from build123d import *

# Parameters (mm, degrees)
EXTRUDE_1_DEPTH = 3


with BuildPart() as part:
    # 草圖1 → 填料-伸長1 (new body)
    with BuildSketch(Plane.XY):
        Polygon((0, -10), (30, -10), (30, -40), (40, -40), (40, -10), (40, 0), (0, 0), align=None)
        Polygon((30, -13.686291501), (26.313708499, -10), (15, -10), (30, -25), align=None)
    extrude(amount=EXTRUDE_1_DEPTH)


solid = part.part
The listing builds one solid part. Answer for the finished solid, in the listing's coordinates (mm). A direction names the side the tool comes from. Coordinates: 2 decimals unless noted, no trailing zeros. Loops run counter-clockwise (first coordinate to the right, second up) from the corner with the lowest first, then second, coordinate; pieces in that order, holes last. Notation, with made-up numbers: (65, 47.5) -> (75, 47.5) arc R18 cw to (75, 61.5) -> close; hole circle Ø10 at (77, -16.5). An arc over 180 degrees is marked (long way). Answer in a Markdown table with one row per item. Add a question column.
1. Consider line 1 (X direction, y = -30.5, z = 1.3); line 2 (Y direction, x = 9, z = 1.7); line 3 (X direction, y = -11, z = 1.3). Determine where each line is inside the solid, lowest interval first. Write a range as [from, to].
2. The part is cut by section C-C, the plane x = 15.5. Write down the section's boundary in (y, z), then the cut area to 3 significant figures.
3. A flat-ended cylindrical pin translates along its axis: P1, Ø0.9, axis at y = -34, z = 2, coming from the -X side. Find the tip coordinate at first contact, or state that the pin passes through.
4. The part is cut by section B-B, the plane y = -28. Write down the section's boundary in (x, z), then the cut area to 3 significant figures.
5. The part is cut by section A-A, the plane z = 1.2. Write down the section's boundary in (x, y).
6. Determine the mould class of faces 4 (the flat face through (0, -5, 1)), 5 (the flat face through (20, 0, 1)), 6 (the flat face through (30, -12, 1)) for opening direction Y: +Y half, -Y half, draft (parallel to the pull), parting line (faces both ways), or undercut.
7. For faces 1 (the flat face through (40, -20, 1)), 2 (the flat face through (7, -10, 1)), 3 (the flat face through (28.183, -11.869, 1.479)), determine the directions among +Z, -Z, +X, -X, +Y, -Y from which every point of the face is accessible in a straight line to the end or side of a thin tool.
Answer below:
| question | item | result |
|---|---|---|
| 1 | line 1 | [30, 40] |
| 1 | line 2 | [-10, 0] |
| 1 | line 3 | [16, 27.31], [30, 40] |
| 2 | outline | (-10.5, 0) -> (0, 0) -> (0, 3) -> (-10.5, 3) -> close |
| 2 | area | 31.5 mm2 |
| 3 | P1 | x = 30 |
| 4 | outline | (30, 0) -> (40, 0) -> (40, 3) -> (30, 3) -> close |
| 4 | area | 30.0 mm2 |
| 5 | outline | (0, -10) -> (15, -10) -> (30, -25) -> (30, -40) -> (40, -40) -> (40, 0) -> (0, 0) -> close; hole (26.31, -10) -> (30, -13.69) -> (30, -10) -> close |
| 6 | face 4 | draft |
| 6 | face 5 | +Y half |
| 6 | face 6 | undercut |
| 7 | face 1 | +Z, -Z, +X, +Y, -Y |
| 7 | face 2 | +Z, -Z, -X, -Y |
| 7 | face 3 | +Z, -Z |
